from build123d import *

# Parameters (mm, degrees)
SKETCH_1_W          = 3
SKETCH_1_H          = 10
SKETCH_1_W_2        = 10
SKETCH_1_H_2        = 3
EXTRUDE_1_DEPTH     = 3
SKETCH_2_W          = 20
SKETCH_2_H          = 20
CUT_EXTRUDE_1_DEPTH = 10
FILLET_1_R          = 3


with BuildPart() as part:
    # 草图1 → 凸台-拉伸1 (new body)
    with BuildSketch(Plane.XY):
        Polygon((-89.861316177, 22.916051468), (-79.861316177, 22.916051468), (-79.861316177, 25.916051468), (-69.861316177, 25.916051468), (-69.861316177, 22.916051468), (-64.861316177, 22.916051468), (-64.861316177, 25.916051468), (-54.861316177, 25.916051468), (-54.861316177, 22.916051468), (-49.861316177, 22.916051468), (-49.861316177, 25.916051468), (-39.861316177, 25.916051468), (-39.861316177, 22.916051468), (-34.861316177, 22.916051468), (-34.861316177, 25.916051468), (-24.861316177, 25.916051468), (-24.861316177, 22.916051468), (-19.861316177, 22.916051468), (-19.861316177, 25.916051468), (-9.861316177, 25.916051468), (-9.861316177, 22.916051468), (-4.861316177, 22.916051468), (-4.861316177, 25.916051468), (5.138683823, 25.916051468), (5.138683823, 22.916051468), (10.138683823, 22.916051468), (10.138683823, 25.916051468), (20.138683823, 25.916051468), (20.138683823, 22.916051468), (25.138683823, 22.916051468), (25.138683823, 25.916051468), (35.138683823, 25.916051468), (35.138683823, 22.916051468), (40.138683823, 22.916051468), (40.138683823, 25.916051468), (50.138683823, 25.916051468), (50.138683823, 22.916051468), (55.138683823, 22.916051468), (55.138683823, 25.916051468), (65.138683823, 25.916051468), (65.138683823, 22.916051468), (70.138683823, 22.916051468), (70.138683823, 25.916051468), (80.138683823, 25.916051468), (80.138683823, 22.916051468), (90.138683823, 22.916051468), (90.138683823, -25.083948532), (-89.861316177, -25.083948532), align=None)
        with Locations((-86.361316177, -0.083948532)):
            Rectangle(SKETCH_1_W, SKETCH_1_H, mode=Mode.SUBTRACT)
        with Locations((-86.361316177, 14.916051468)):
            Rectangle(SKETCH_1_W, SKETCH_1_H, mode=Mode.SUBTRACT)
        with Locations((-86.361316177, -15.083948532)):
            Rectangle(SKETCH_1_W, SKETCH_1_H, mode=Mode.SUBTRACT)
        with Locations((86.638683823, -15.083948532)):
            Rectangle(SKETCH_1_W, SKETCH_1_H, mode=Mode.SUBTRACT)
        with Locations((86.638683823, -0.083948532)):
            Rectangle(SKETCH_1_W, SKETCH_1_H, mode=Mode.SUBTRACT)
        with Locations((86.638683823, 14.916051468)):
            Rectangle(SKETCH_1_W, SKETCH_1_H, mode=Mode.SUBTRACT)
        with Locations((-59.861316177, -21.583948532)):
            Rectangle(SKETCH_1_W_2, SKETCH_1_H_2, mode=Mode.SUBTRACT)
        with Locations((-74.861316177, -21.583948532)):
            Rectangle(SKETCH_1_W_2, SKETCH_1_H_2, mode=Mode.SUBTRACT)
        with Locations((-44.861316177, -21.583948532)):
            Rectangle(SKETCH_1_W_2, SKETCH_1_H_2, mode=Mode.SUBTRACT)
        with Locations((-29.861316177, -21.583948532)):
            Rectangle(SKETCH_1_W_2, SKETCH_1_H_2, mode=Mode.SUBTRACT)
        with Locations((-14.861316177, -21.583948532)):
            Rectangle(SKETCH_1_W_2, SKETCH_1_H_2, mode=Mode.SUBTRACT)
        with Locations((0.138683823, -21.583948532)):
            Rectangle(SKETCH_1_W_2, SKETCH_1_H_2, mode=Mode.SUBTRACT)
        with Locations((15.138683823, -21.583948532)):
            Rectangle(SKETCH_1_W_2, SKETCH_1_H_2, mode=Mode.SUBTRACT)
        with Locations((30.138683823, -21.583948532)):
            Rectangle(SKETCH_1_W_2, SKETCH_1_H_2, mode=Mode.SUBTRACT)
        with Locations((45.138683823, -21.583948532)):
            Rectangle(SKETCH_1_W_2, SKETCH_1_H_2, mode=Mode.SUBTRACT)
        with Locations((60.138683823, -21.583948532)):
            Rectangle(SKETCH_1_W_2, SKETCH_1_H_2, mode=Mode.SUBTRACT)
        with Locations((75.138683823, -21.583948532)):
            Rectangle(SKETCH_1_W_2, SKETCH_1_H_2, mode=Mode.SUBTRACT)
    extrude(amount=EXTRUDE_1_DEPTH)

    # 草图2 → 切除-拉伸1 (cut)
    with BuildSketch(Plane.XY.offset(3)):
        with Locations((65.138683823, 1.413515523)):
            Rectangle(SKETCH_2_W, SKETCH_2_H)
        with Locations((-65.138683823, 1.413515523)):
            Rectangle(SKETCH_2_W, SKETCH_2_H)
    extrude(amount=-CUT_EXTRUDE_1_DEPTH, mode=Mode.SUBTRACT)

    # 圆角1
    fillet_1_edges = [part.edges().sort_by_distance(p)[0] for p in [
        (75.138683823, 11.413515523, 1.5),
        (75.138683823, -8.586484477, 1.5),
        (55.138683823, -8.586484477, 1.5),
        (55.138683823, 11.413515523, 1.5),
        (-55.138683823, 11.413515523, 1.5),
        (-55.138683823, -8.586484477, 1.5),
        (-75.138683823, -8.586484477, 1.5),
        (-75.138683823, 11.413515523, 1.5),
    ]]
    fillet(fillet_1_edges, radius=FILLET_1_R)


solid = part.part
Design review of the part built by this model. Coordinates are the model's own, in mm. A direction names the side the tool comes from. Give positions to 0.01 mm unless a question says otherwise; leave off trailing zeros. Write each loop counter-clockwise with the first axis right and the second up, starting at its lowest first coordinate (ties: lowest second). Pieces come first, ordered by that corner, then holes. Notation, with made-up numbers: M 0.5,69 L 53.5,69 A23 cw 53.5,82 Z; hole C -20.5,5.25 d6. An arc over 180 degrees is marked long. Answer as a JSON object with one key per item and string values. Group by question number.
1) We need section D-D (z = 2.05). Count the separate pieces of the cut face and the enclosed holes in it, and give its area (3 significant figures).
2) We need section A-A (y = -2). Give the boundary of the cut face in (x, z), and give its area (3 significant figures).
3) Tool access review of faces 4 (the face through (-19.861, 24, 1)), 5 (the face through (80.139, 24, 1)), 6 (the face through (-65, 11.414, 2)): name each direction out of +Z, -Z, +X, -X, +Y, -Y from which nothing blocks a thin tool from reaching the whole face with its end or side.
4) We need section B-B (x = -32). Give the boundary of the cut face in (y, z), and give its area (3 significant figures).
5) For line 1 along X through (y, z) = (8, 1.85); line 2 along X through (y, z) = (-1.5, 0.2); line 3 along X through (y, z) = (11.5, 1.6), list the stretches that pass through material, from the lowest coordinate up.
6) We need section C-C (y = -16). Give the boundary of the cut face in (x, z), and give its area (3 significant figures).
7) Clearance check with a flat-ended pin moving along its axis: pin 1 Ø1.5 at (x, z) = (-51, 1) entering from +Y. State where the tip first meets the part, or that it passes through.
8) Mouldability with a two-part tool opening along Y and no side actions: class faces 1 (the face through (87, 9.916, 1)), 2 (the face through (45, 25.916, 1)), 3 (the face through (1, 1, 3)) as released by +Y, released by -Y, zero draft, split by the parting line, or undercut.
Answer key:
{
 "1": {"separate pieces": "1", "enclosed holes": "19", "area": "7,680 mm²"},
 "2": {"outline": "M -89.86,0 L -87.86,0 L -87.86,3 L -89.86,3 Z; M -84.86,0 L -75.14,0 L -75.14,3 L -84.86,3 Z; M -55.14,0 L 55.14,0 L 55.14,3 L -55.14,3 Z; M 75.14,0 L 85.14,0 L 85.14,3 L 75.14,3 Z; M 88.14,0 L 90.14,0 L 90.14,3 L 88.14,3 Z", "area": "402 mm²"},
 "3": {"face 4": "+Z, -Z, +Y", "face 5": "+Z, -Z, +X, +Y", "face 6": "+Z, -Z"},
 "4": {"outline": "M -25.08,0 L -23.08,0 L -23.08,3 L -25.08,3 Z; M -20.08,0 L 25.92,0 L 25.92,3 L -20.08,3 Z", "area": "144 mm²"},
 "5": {"line 1": "x = -89.86 to -75.14, -55.14 to 55.14, 75.14 to 90.14", "line 2": "x = -89.86 to -87.86, -84.86 to -75.14, -55.14 to 55.14, 75.14 to 85.14, 88.14 to 90.14", "line 3": "x = -89.86 to -87.86, -84.86 to 85.14, 88.14 to 90.14"},
 "6": {"outline": "M -89.86,0 L -87.86,0 L -87.86,3 L -89.86,3 Z; M -84.86,0 L 85.14,0 L 85.14,3 L -84.86,3 Z; M 88.14,0 L 90.14,0 L 90.14,3 L 88.14,3 Z", "area": "522 mm²"},
 "7": {"pin 1": "stops at y = 22.92"},
 "8": {"face 1": "undercut", "face 2": "released by +Y", "face 3": "zero draft"}
}
